The listing builds one solid part. Answer for the finished solid, in the listing's coordinates (mm). Face numbers are marked on the shaded views. Give positions to 0.01 mm unless a question says otherwise; leave off trailing zeros. Loops run counter-clockwise (first coordinate to the right, second up) from the corner with the lowest first, then second, coordinate; pieces in that order, holes last. Notation, with made-up numbers: (68.25, 16) - (78.25, 16) arc R22 cw to (78.25, 24) - close; hole circle Ø8 at (87, 85). An arc over 180 degrees is marked (long way). One line per item, written item: value. Start each with the question number.
Autodesk Inventor part; units mm, degrees
ref_plane "YZ Plane" through (0, 0, 0) normal (1, 0, 0) x (0, 1, 0)
ref_plane "XZ Plane" through (0, 0, 0) normal (0, 1, 0) x (-1, 0, 0)
ref_plane "XY Plane" through (0, 0, 0) normal (0, 0, 1) x (1, 0, 0)
sketch "スケッチ1" plane through (0, 0, 0) normal (0, 0, 1) x (1, 0, 0)
  circle A0 centre (0, 0) radius 45
  circle A1 centre (0, 0) radius 57.5
  dimension "d0" = 90
  dimension "d1" = 115
extrude "押し出し1" add sketch "スケッチ1" along normal blind 8.5
sketch "スケッチ2" plane through (0, 0, 8.5) normal (0, 0, 1) x (1, 0, 0)
  line L0 (0, 0) -> (35.7, 0)
  line L1 (35.7, 0) -> (35.7, -35.7)
  line L2 (35.7, -35.7) -> (0, -35.7)
  line L3 (0, -35.7) -> (0, 0)
  point P0 (35.7, 35.7)
  point P1 (-35.7, 35.7)
  point P2 (-35.7, -35.7)
  dimension "d13" = 35.7
  dimension "d14" = 35.7
  dimension "d17" = 360
hole "穴1" at (-35.7, 35.7, 8.5) at (35.7, 35.7, 8.5) at (-35.7, -35.7, 8.5) at (35.7, -35.7, 8.5) direction (0, 0, -1) diameter 5 end through all
fillet "フィレット1" radius 1 2 edges at (-45, 0, 8.5) (-57.5, 0, 8.5)
properties part number "turntable_in_8_23" material "アルミニウム 6061-AHC"
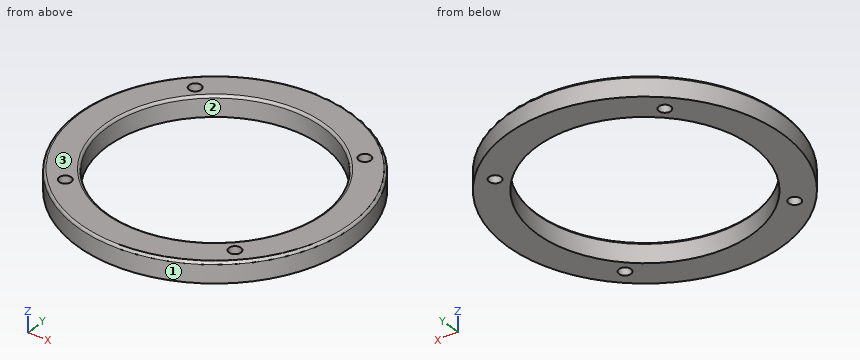
1. A cutting plane is placed at D-D (y = 35.7). Give the number of separate pieces and of enclosed holes in the cut face, plus the area to 3 significant figures.
2. Flat-ended cylindrical pins translate along their axes: pin 1 (1 mm diameter, centred on y = -28.5, z = 3.5, fed in from +X); pin 2 (3 mm diameter, centred on y = 24.5, z = 6.5, fed in from +X); pin 3 (2 mm diameter, centred on y = 20.5, z = 7, fed in from -X); pin 4 (4.5 mm diameter, centred on x = -35.7, y = 35.7, fed in from -Z). Find the tip coordinate at first contact, or state that the pin passes through.
3. Find the intervals of material crossed by L1, parallel to X at y = -35.7, z = 4.5; L2, parallel to Y at x = -41, z = 5.25, in increasing order. Write a range as [from, to].
4. A cutting plane is placed at A-A (y = 0). Determine the outline of the cut face in (x, z).
5. A cutting plane is placed at B-B (z = 5.25). Determine the outline of the cut face in (x, y), plus the area to 3 significant figures.
6. Determine the mould class of the marked faces 1, 2 and 3 for opening direction Y: released by +Y, released by -Y, zero draft, split by the parting line, or undercut.
Results below:
1. separate pieces: 4
1. enclosed holes: 0
1. area: 214 mm^2
2. pin 1: stops at x = 50.22
2. pin 2: stops at x = 52.7
2. pin 3: stops at x = -54.09
2. pin 4: passes through
3. L1: x = [-45.08, -38.2], [-33.2, -27.4], [27.4, 33.2], [38.2, 45.08]
3. L2: y = [-40.31, -18.55], [18.55, 40.31]
4. outline: (-57.5, 0) - (-45, 0) - (-45, 7.5) arc R1 ccw to (-46, 8.5) - (-56.5, 8.5) arc R1 ccw to (-57.5, 7.5) - close; (45, 0) - (57.5, 0) - (57.5, 7.5) arc R1 ccw to (56.5, 8.5) - (46, 8.5) arc R1 ccw to (45, 7.5) - close
5. outline: circle Ø115 at (0, 0); hole circle Ø90 at (0, 0); hole circle Ø5 at (-35.7, -35.7); hole circle Ø5 at (-35.7, 35.7); hole circle Ø5 at (35.7, -35.7); hole circle Ø5 at (35.7, 35.7)
5. area: 3,950 mm^2
6. face 1: split by the parting line
6. face 2: undercut
6. face 3: zero draft
